from build123d import *

# Parameters (mm, degrees)
SKETCH1_W           = 38.1
SKETCH1_H           = 391.16
BOSS_EXTRUDE1_DEPTH = 4.064
SKETCH2_R           = 10
CUT_EXTRUDE1_DEPTH  = 3.863999892
BOSS_EXTRUDE2_DEPTH = 4.064


with BuildPart() as part:
    # Sketch1 → Boss-Extrude1 (new body)
    with BuildSketch(Plane(origin=(0, 0, 0), x_dir=(1, 0, 0), z_dir=(0, 1, 0))):
        Rectangle(SKETCH1_W, SKETCH1_H)
    extrude(amount=BOSS_EXTRUDE1_DEPTH)

    # Sketch2 → Cut-Extrude1 (cut)
    with BuildSketch(Plane(origin=(0, 4.064, 0), x_dir=(1, 0, 0), z_dir=(0, 1, 0))):
        with Locations(Location((0, 177.8, 0), (0, 0, 270))):
            Circle(SKETCH2_R)
        with Locations(Location((0, 152.4, 0), (0, 0, 270))):
            Circle(SKETCH2_R)
        with Locations(Location((0, 127, 0), (0, 0, 270))):
            Circle(SKETCH2_R)
        with Locations(Location((0, 101.6, 0), (0, 0, 270))):
            Circle(SKETCH2_R)
        with Locations(Location((0, 76.2, 0), (0, 0, 270))):
            Circle(SKETCH2_R)
        with Locations(Location((0, 50.8, 0), (0, 0, 270))):
            Circle(SKETCH2_R)
        with Locations(Location((0, 25.4, 0), (0, 0, 270))):
            Circle(SKETCH2_R)
        with Locations(Location((0, 0, 0), (0, 0, 270))):
            Circle(SKETCH2_R)
        with Locations(Location((0, -25.4, 0), (0, 0, 270))):
            Circle(SKETCH2_R)
        with Locations(Location((0, -50.8, 0), (0, 0, 270))):
            Circle(SKETCH2_R)
        with Locations(Location((0, -76.2, 0), (0, 0, 270))):
            Circle(SKETCH2_R)
        with Locations(Location((0, -101.6, 0), (0, 0, 270))):
            Circle(SKETCH2_R)
        with Locations(Location((0, -127, 0), (0, 0, 270))):
            Circle(SKETCH2_R)
        with Locations(Location((0, -152.4, 0), (0, 0, 270))):
            Circle(SKETCH2_R)
        with Locations(Location((0, -177.8, 0), (0, 0, 270))):
            Circle(SKETCH2_R)
    extrude(amount=-CUT_EXTRUDE1_DEPTH, mode=Mode.SUBTRACT)

    # Sketch4 → Boss-Extrude2 (add)
    with BuildSketch(Plane(origin=(0, 0, 0), x_dir=(1, 0, 0), z_dir=(0, 1, 0))):
        Polygon((28.482303355, -55.490633493), (19.05, -56.81625728), (19.05, -73.215009707), (28.482303355, -74.540633493), align=None)
        Polygon((28.482303355, 146.105623787), (19.05, 144.78), (19.05, 128.381247573), (28.482303355, 127.055623787), align=None)
        Polygon((-19.05, 128.381247573), (-19.05, 144.78), (-28.482303355, 146.105623787), (-28.482303355, 127.055623787), align=None)
        Polygon((28.482303355, 78.90687136), (19.05, 77.581247573), (19.05, 61.182495147), (28.482303355, 59.85687136), align=None)
        Polygon((28.482303355, 11.708118933), (19.05, 10.382495147), (19.05, -6.01625728), (28.482303355, -7.341881067), align=None)
        Polygon((-19.05, -6.01625728), (-19.05, 10.382495147), (-28.482303355, 11.708118933), (-28.482303355, -7.341881067), align=None)
        Polygon((-19.05, 61.182495147), (-19.05, 77.581247573), (-28.482303355, 78.90687136), (-28.482303355, 59.85687136), align=None)
        Polygon((28.482303355, -122.68938592), (19.05, -124.015009707), (19.05, -140.413762134), (28.482303355, -141.73938592), align=None)
        Polygon((-19.05, -140.413762134), (-19.05, -124.015009707), (-28.482303355, -122.68938592), (-28.482303355, -141.73938592), align=None)
        Polygon((-19.05, -73.215009707), (-19.05, -56.81625728), (-28.482303355, -55.490633493), (-28.482303355, -74.540633493), align=None)
    extrude(amount=BOSS_EXTRUDE2_DEPTH)


solid = part.part
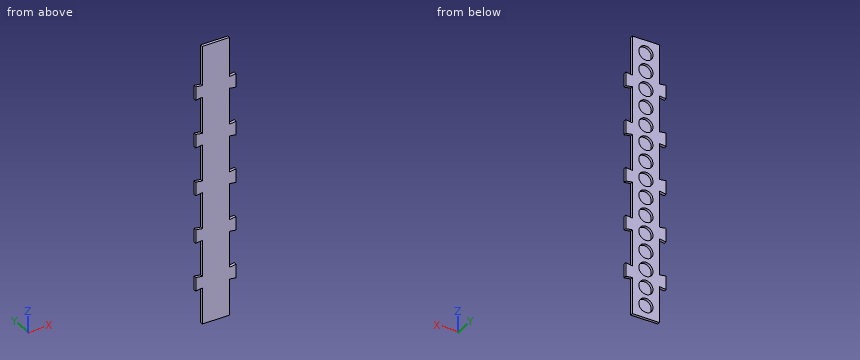
Verification items for the finished model (mm, model axes). Coordinates: 2 decimals unless noted, no trailing zeros. Write each loop counter-clockwise with the first axis right and the second up, starting at its lowest first coordinate (ties: lowest second). Pieces come first, ordered by that corner, then holes. Notation, with made-up numbers: (81.25, 14) - (85.25, 14) arc R27 cw to (85.25, 39) - close; hole circle Ø10 at (-39.5, 51). An arc over 180 degrees is marked (long way). Answer as a JSON object with one key per item and string values.
(1) Cross-section at B-B on x = -23. Record the cut outline in (y, z).
Report:
{"outline": "(0, -145.34) - (4.06, -145.34) - (4.06, -127.83) - (0, -127.83) - close; (0, -78.14) - (4.06, -78.14) - (4.06, -60.63) - (0, -60.63) - close; (0, -10.94) - (4.06, -10.94) - (4.06, 6.57) - (0, 6.57) - close; (0, 56.26) - (4.06, 56.26) - (4.06, 73.77) - (0, 73.77) - close; (0, 123.46) - (4.06, 123.46) - (4.06, 140.97) - (0, 140.97) - close"}
(2) Cross-section at C-C on y = 2.8. Give the number of separate pieces and of enclosed holes in the cut face, plus the area to 3 significant figures.
Report:
{"separate pieces": "1", "enclosed holes": "15", "area": "11,900 mm^2"}
(3) Cross-section at A-A on z = 152.4. Record the cut outline in (x, y).
Report:
{"outline": "(-19.05, 0) - (19.05, 0) - (19.05, 4.06) - (10, 4.06) - (10, 0.2) - (-10, 0.2) - (-10, 4.06) - (-19.05, 4.06) - close"}
(4) Thickness scan on line 1 along Z through (x, y) = (-23, 3.25); line 2 along X through (y, z) = (1.1, 127); line 3 along X through (y, z) = (1.75, -177.8). Record the ranges inside material, lowest first.
Report:
{"line 1": "-145.34 to -127.83, -78.14 to -60.63, -10.94 to 6.57, 56.26 to 73.77, 123.46 to 140.97", "line 2": "-28.48 to -10, 10 to 28.48", "line 3": "-19.05 to -10, 10 to 19.05"}
(5) Gauge pin test, flat ends, axial feed: pin 1 Ø6 at (x, z) = (4, 80.5) entering from +Y; pin 2 Ø1.2 at (y, z) = (1.5, -180.5) entering from +X; pin 3 Ø1.5 at (x, y) = (-22.5, 2.5) entering from +Z. Record the tip position at first contact, or that the pin passes through.
Report:
{"pin 1": "y = 0.2", "pin 2": "x = 19.05", "pin 3": "z = 141"}
